Autodesk Inventor part; units mm, degrees
ref_plane "YZ Plane" through (0, 0, 0) normal (1, 0, 0) x (0, 1, 0)
ref_plane "XZ Plane" through (0, 0, 0) normal (0, 1, 0) x (-1, 0, 0)
ref_plane "XY Plane" through (0, 0, 0) normal (0, 0, 1) x (1, 0, 0)
sketch "スケッチ1" plane through (0, 0, 0) normal (1, 0, 0) x (0, 1, 0)
  line L0 (0, 0) -> (45, 0)
  line L1 (45, 0) -> (45, 15)
  line L2 (45, 15) -> (0, 15)
  line L3 (0, 15) -> (0, 0)
  line L4 (0, 0) -> (15, 0)
  line L5 (15, 0) -> (15, 30)
  line L6 (15, 30) -> (0, 30)
  line L7 (0, 30) -> (0, 0)
  point P0 (0, 15)
  point P1 (15, 15)
  dimension "d0" = 15
  dimension "d1" = 15
  dimension "d2" = 30
  dimension "d3" = 30
extrude "押し出し1" add sketch "スケッチ1" along normal blind 2
sketch "スケッチ2" plane through (2, 0, 0) normal (1, 0, 0) x (0, 0, -1)
  line L0 (-30, 15) -> (-30, 0)
  line L1 (-30, 7.5) -> (0, 7.5) construction
  line L2 (0, 0) -> (0, 45)
  line L3 (0, 45) -> (-15, 45)
  line L4 (-7.5, 45) -> (-7.5, 0) construction
  line L5 (-30, 0) -> (0, 0)
  point P0 (-25, 7.5)
  point P1 (-5, 7.5)
  point P2 (-7.5, 20)
  point P3 (-7.5, 40)
  dimension "d6" = 20
  dimension "d7" = 5
  dimension "d8" = 20
  dimension "d9" = 5
hole "穴1" at (2, 7.5, 25) at (2, 7.5, 5) at (2, 20, 7.5) at (2, 40, 7.5) direction (-1, 0, 0) diameter 3.2 end through all
properties part number "FrameJointL1515" material "アルミニウム 6061"
Verification items for the finished model (mm, model axes). A direction names the side the tool comes from. Round coordinates to 2 decimals unless told otherwise and drop trailing zeros. Write each loop counter-clockwise with the first axis right and the second up, starting at its lowest first coordinate (ties: lowest second). Pieces come first, ordered by that corner, then holes.
(1) Material ranges on line 1 (Z direction, x = 1.5, y = 7.5); line 2 (Y direction, x = 1.3, z = 7.5); line 3 (Y direction, x = 0.8, z = 25), recorded low to high.
Returned:
line 1: z = 0 to 3.4, 6.6 to 23.4, 26.6 to 30
line 2: y = 0 to 18.4, 21.6 to 38.4, 41.6 to 45
line 3: y = 0 to 5.9, 9.1 to 15
(2) Section check A-A (z = 7.5). Enter the section's corners in (x, y).
Returned:
outline: (0, 0) - (2, 0) - (2, 18.4) - (0, 18.4) - close; (0, 21.6) - (2, 21.6) - (2, 38.4) - (0, 38.4) - close; (0, 41.6) - (2, 41.6) - (2, 45) - (0, 45) - close
(3) Section check C-C (x = 1.6). Enter the section's corners in (y, z).
Returned:
outline: (0, 0) - (45, 0) - (45, 15) - (15, 15) - (15, 30) - (0, 30) - close; hole circle Ø3.2 at (7.5, 5); hole circle Ø3.2 at (7.5, 25); hole circle Ø3.2 at (20, 7.5); hole circle Ø3.2 at (40, 7.5)
(4) Mould release check, pull along Y, two halves, no side actions. Record for faces 3 (the cylindrical face through (0.986, 18.414, 7.708)), 4 (the flat face through (1, 0, 15)), 5 (the cylindrical face through (0.99, 41.42, 6.76)), 6 (the flat face through (1, 30, 15)): pulls with the +Y half, pulls with the -Y half, needs draft (parallel to the pull), parting line crosses it, or undercut.
Returned:
face 3: undercut
face 4: pulls with the -Y half
face 5: undercut
face 6: needs draft
(5) Section check D-D (y = 25.5). Enter the section's corners in (x, z), plus the area to 3 significant figures.
Returned:
outline: (0, 0) - (2, 0) - (2, 15) - (0, 15) - close
area: 30.0 mm2
(6) Section check B-B (y = 20). Enter the section's corners in (x, z), plus the area to 3 significant figures.
Returned:
outline: (0, 0) - (2, 0) - (2, 5.9) - (0, 5.9) - close; (0, 9.1) - (2, 9.1) - (2, 15) - (0, 15) - close
area: 23.6 mm2
(7) Access from +Z, -Z, +X, -X, +Y, -Y to the whole of each face (thin tool, end or side, straight path). Record for faces 1 (the flat face through (1, 15, 22)), 2 (the flat face through (2, 17, 12)).
Returned:
face 1: +Z, +X, -X, +Y
face 2: +Z, -Z, +X, +Y, -Y
(8) Depth check by flat-ended pin: pin 1 Ø2.5 at (y, z) = (7.5, 25) entering from +X. Enter the tip coordinate at first touch or a pass-through.
Returned:
pin 1: passes through
